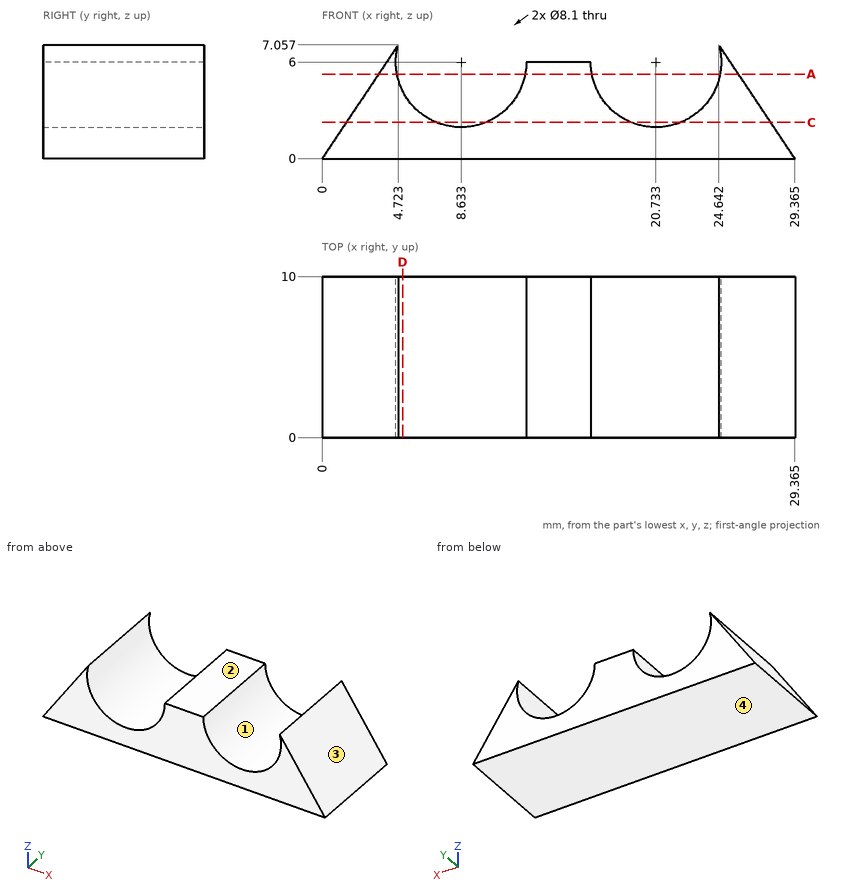
Input: dimensioned drawing with shaded views. Units: mm. Origin: part minimum x, y, z. Give positions to 0.01 mm unless a question says otherwise; leave off trailing zeros. Write each loop counter-clockwise with the first axis right and the second up, starting at its lowest first coordinate (ties: lowest second). Pieces come first, ordered by that corner, then holes.
1. Pin query (flat end, axial travel): P1, Ø2, axis at y = 1.5, z = 3, coming from the +X side; P2, Ø4.5, axis at x = 15, y = 6.5, coming from the +Z side. Return the tip coordinate at first contact, or that it passes through.
2. Line query: probe 1 along X at (y, z) = (5.5, 4.5) (1 decimal); probe 2 along X at (y, z) = (8.5, 4.25) (1 decimal); probe 3 along Z at (x, y) = (8.5, 7). Output: solid intervals per line, ascending.
3. Section query C-C, the plane z = 2.25. Return loops of the section in (x, y) (1 decimal), then the cut area to 3 significant figures.
4. Draft query along X for the marked faces 1, 2, 3 and 4. Return one class per face: released by +X, released by -X, zero draft, split by the parting line, or undercut.
5. Section query A-A, the plane z = 5.25. Return loops of the section in (x, y).
6. Section query D-D, the plane x = 5. Return loops of the section in (y, z).
Computed:
1. P1: stops at x = 28.03
1. P2: stops at z = 6
2. probe 1: x = 3 to 4.9, 12.4 to 17, 24.5 to 26.4
2. probe 2: x = 2.8 to 5, 12.3 to 17.1, 24.4 to 26.5
2. probe 3: z = 0 to 1.95
3. outline: (1.5, 0) - (7.1, 0) - (7.1, 10) - (1.5, 10) - close; (10.2, 0) - (19.2, 0) - (19.2, 10) - (10.2, 10) - close; (22.3, 0) - (27.9, 0) - (27.9, 10) - (22.3, 10) - close
3. area: 202 mm2
4. face 1: undercut
4. face 2: undercut
4. face 3: released by +X
4. face 4: zero draft
5. outline: (3.51, 0) - (4.65, 0) - (4.65, 10) - (3.51, 10) - close; (12.61, 0) - (16.75, 0) - (16.75, 10) - (12.61, 10) - close; (24.71, 0) - (25.85, 0) - (25.85, 10) - (24.71, 10) - close
6. outline: (0, 0) - (10, 0) - (10, 4.21) - (0, 4.21) - close
